from build123d import *

# Parameters (mm, degrees)
F0_R     = 11.5
F0_R_2   = 10.25
F1_DEPTH = 20
F2_R     = 22.5
F3_DEPTH = 15
F4_R     = 12
F5_R     = 2.99999


# Not quite as in the source:
# - a fillet or chamfer is up to 0.001 mm smaller than in the source, because OpenCascade refuses the exact size


with BuildPart() as f1:
    # F0 (on Front) → F1 (new body)
    with BuildSketch(Plane.XZ):
        Circle(F0_R)
        Circle(F0_R_2, mode=Mode.SUBTRACT)
    extrude(amount=F1_DEPTH)

    # F2 (on face) → F3 (join)
    with BuildSketch(Plane.XZ.offset(20)):
        Circle(F2_R)
    extrude(amount=F3_DEPTH)

    # F4
    f4_edges = [f1.edges().sort_by_distance(p)[0] for p in [
        (-22.5, -35, 0),
    ]]
    fillet(f4_edges, radius=F4_R)

    # F5 (radius 3 in the source; OpenCascade refuses exactly that, so slightly less here)
    f5_edges = [f1.edges().sort_by_distance(p)[0] for p in [
        (-10.5, -35, 0),
        (-22.5, -23, 0),
        (-22.5, -20, 0),
    ]]
    fillet(f5_edges, radius=F5_R)


solid = f1.part
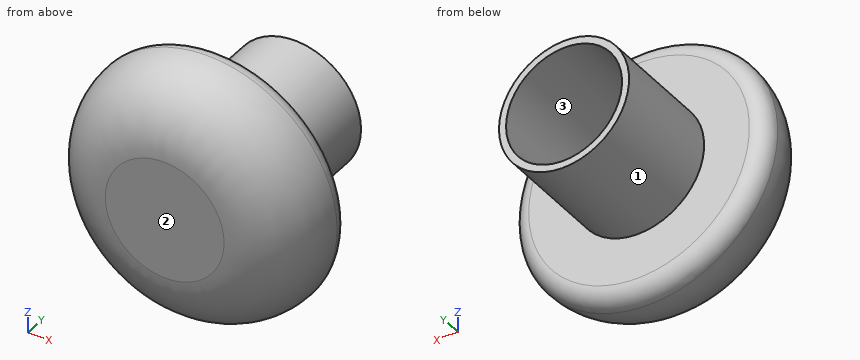
Here's how the part is built. I have some questions about the finished solid (model axes, mm). Face numbers are marked on the shaded views. Give positions to 0.01 mm unless a question says otherwise; leave off trailing zeros. Loops run counter-clockwise (first coordinate to the right, second up) from the corner with the lowest first, then second, coordinate; pieces in that order, holes last. Notation, with made-up numbers: (-35, -29) -> (-25, -29) arc R15 cw to (-25, -24) -> close; hole circle Ø1 at (-9, 38.5). An arc over 180 degrees is marked (long way). Answer as a JSON object with one key per item and string values. Group by question number.
Item 1: Thinking about a two-plate mould opening in Z: for the marked faces 1, 2 and 3, which applies, pulls with the +Z half, pulls with the -Z half, needs draft (parallel to the pull), parting line crosses it, or undercut?
Item 2: I need wall thicknesses on L1, parallel to X at y = -3.5, z = -1; L2, parallel to X at y = -6, z = -9.5; L3, parallel to Z at x = 8.5, y = -7. Which ranges of each line are inside material? Lowest first, please.
Item 3: Will these pins go through, and if not, where does the flat tip stop? pin 1 (1 mm diameter, centred on x = 8, y = -22, fed in from +Z); pin 2 (12 mm diameter, centred on y = -4, z = 15.5, fed in from -X); pin 3 (10 mm diameter, centred on x = 14.5, z = -14.5, fed in from -Y).
Item 4: Imagine slicing it at A-A on y = -9. Write out the boundary of the cut face in (x, z), then the cut area to 3 significant figures.
Answer list:
{
 "1": {"face 1": "parting line crosses it", "face 2": "needs draft", "face 3": "undercut"},
 "2": {"L1": "x = -11.46 to -10.2, 10.2 to 11.46", "L2": "x = -6.48 to -3.85, 3.85 to 6.48", "L3": "z = -7.75 to -5.73, 5.73 to 7.75"},
 "3": {"pin 1": "stops at z = 21.09", "pin 2": "stops at x = -6.48", "pin 3": "stops at y = -33.91"},
 "4": {"outline": "circle Ø23 at (0, 0); hole circle Ø20.5 at (0, 0)", "area": "85.4 mm2"}
}
